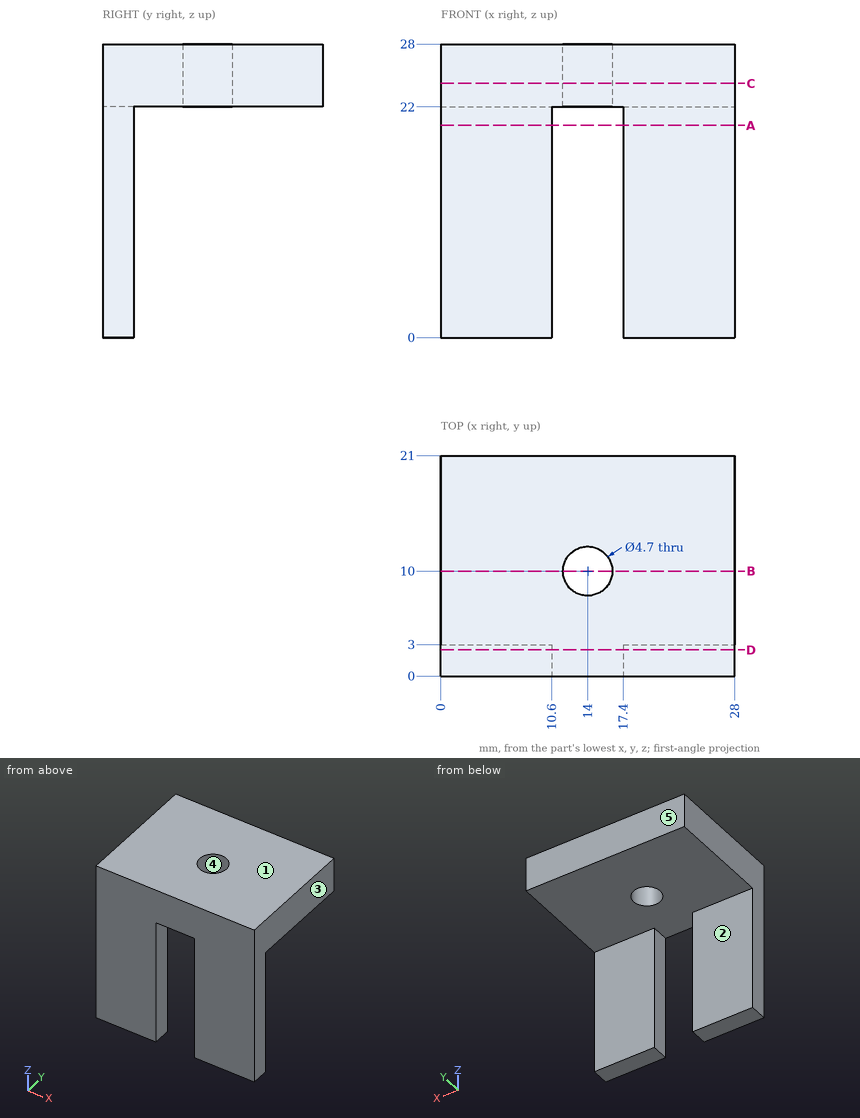
Source: three-view drawing plus pictorial views. Frame: mm from the lowest corner of the part. A direction names the side the tool comes from. Round coordinates to 2 decimals unless told otherwise and drop trailing zeros. Order: outer loops, then holes, each group sorted by start corner. A loop starts at its lowest first (then second) coordinate and runs counter-clockwise, first axis right, second up. Notation, with made-up numbers: (13.5, 60) -> (48.5, 60) arc R12 ccw to (48.5, 69) -> close; hole circle Ø3 at (80.5, 69.5). An arc over 180 degrees is marked (long way). Use one line per item in the form item = value.
(1) Access query for the marked faces 1 and 2. Directions: +Z, -Z, +X, -X, +Y, -Y. A direction counts if a zero-diameter tool reaches every point of the face in a straight line with its end or side. Return the directions, or none.
Results list:
face_1 = +Z, +X, -X, +Y, -Y
face_2 = -Z, +X, -X, +Y
(2) Section B-B on y = 10. Return loops of the section in (x, z).
Results list:
outline = (0, 22) -> (11.65, 22) -> (11.65, 28) -> (0, 28) -> close; (16.35, 22) -> (28, 22) -> (28, 28) -> (16.35, 28) -> close
(3) Draft query along X for the marked faces 3, 4 and 5. Return one class per face: pulls with the +X half, pulls with the -X half, needs draft (parallel to the pull), parting line crosses it, or undercut.
Results list:
face_3 = pulls with the +X half
face_4 = undercut
face_5 = needs draft
(4) Section D-D on y = 2.5. Return loops of the section in (x, z), and give its area (3 significant figures).
Results list:
outline = (0, 0) -> (10.6, 0) -> (10.6, 22) -> (17.4, 22) -> (17.4, 0) -> (28, 0) -> (28, 28) -> (0, 28) -> close
area = 634 mm^2
(5) Section A-A on z = 20.25. Return loops of the section in (x, y), and give its area (3 significant figures).
Results list:
outline = (0, 0) -> (10.6, 0) -> (10.6, 3) -> (0, 3) -> close; (17.4, 0) -> (28, 0) -> (28, 3) -> (17.4, 3) -> close
area = 63.6 mm^2
(6) Section C-C on z = 24.25. Return loops of the section in (x, y), and give its area (3 significant figures).
Results list:
outline = (0, 0) -> (28, 0) -> (28, 21) -> (0, 21) -> close; hole circle Ø4.7 at (14, 10)
area = 571 mm^2
(7) Ray query, probe 1 along Y at (x, z) = (14, 25.15); probe 2 along Z at (x, y) = (22, 17.75); probe 3 along Y at (x, z) = (9.5, 20). Return the intervals inside material, ascending. Write a range as [from, to].
Results list:
probe_1 = [0, 7.65], [12.35, 21]
probe_2 = [22, 28]
probe_3 = [0, 3]
(8) First-contact query: pin 1 Ø5 at (x, z) = (9.5, 16) entering from +Y; pin 2 Ø4 at (x, y) = (14, 10) entering from +Z; pin 3 Ø1 at (x, y) = (12.5, 2.5) entering from -Z. Flat tips, straight axial feed; report the tip coordinate or a pass-through.
Results list:
pin_1 = 3
pin_2 = through
pin_3 = 22
